CAD build for the part. Positions are in the model's coordinates, mm. A direction names the side the tool comes from. Give positions to 0.01 mm unless a question says otherwise; leave off trailing zeros. Order: outer loops, then holes, each group sorted by start corner. A loop starts at its lowest first (then second) coordinate and runs counter-clockwise, first axis right, second up.
Item 1: Band-saw the part on C-C on z = 0. Count the separate pieces of the cut face and the enclosed holes in it, plus the area to 3 significant figures.
Item 2: Wall check: L1, parallel to Z at x = -762, y = 481; L2, parallel to Y at x = -149, z = -17.5; L3, parallel to X at y = -95, z = 24.5. Give the ranges that are in metal, low to high.
Item 3: Band-saw the part on A-A on x = 762. Give the cut face in (y, z).
Item 4: Band-saw the part on B-B on y = -310. Give the cut face in (x, z).
Item 5: Two-plate mould, pull along Z, no slides. Class faces 1 (the flat face through (1016, -7, 3)), 2 (the cylindrical face through (-825.44, -476.69, 2.79)), 3 (the flat face through (-80, -449, 190.5)): released by +Z, released by -Z, zero draft, split by the parting line, or undercut.
Item 6: Band-saw the part on D-D on x = -408. Give the cut face in (y, z), plus the area to 3 significant figures.
Item 7: Which spindle directions (+Z, -Z, +X, -X, +Y, -Y) get a long thin tool onto all of the face, cutting with end or side? Do faces 4 (the flat face through (-952.5, -6, 3)), 5 (the cylindrical face through (825.44, -476.69, -2.79)). Say none if no direction does.
```python
from build123d import *

# Parameters (mm, degrees)
F0_W     = 2032
F0_H     = 1016
F0_W_2   = 1905
F0_H_2   = 889
F1_DEPTH = 190.5
F2_R     = 63.5
F3_DEPTH = 1016.001


with BuildPart() as f1:
    # F0 (on Top) → F1 (new body, symmetric)
    with BuildSketch(Plane.XY):
        Rectangle(F0_W, F0_H)
        Rectangle(F0_W_2, F0_H_2, mode=Mode.SUBTRACT)
    extrude(amount=F1_DEPTH, both=True)

    # F2 (on face) → F3 (cut, through all)
    with BuildSketch(Plane.XZ.offset(508)):
        with BuildLine():
            ThreePointArc((825.5, 0), (762, 63.5), (698.5, 0))
            ThreePointArc((698.5, 0), (762, -63.5), (825.5, 0))
        make_face()
        with BuildLine():
            ThreePointArc((63.5, 0), (0, 63.5), (-63.5, 0))
            Line((-63.5, 0), (63.5, 0))
        make_face()
        with BuildLine():
            Line((63.5, 0), (-63.5, 0))
            ThreePointArc((-63.5, 0), (0, -63.5), (63.5, 0))
        make_face()
        with Locations((-762, 0)):
            Circle(F2_R)
    extrude(amount=-F3_DEPTH, mode=Mode.SUBTRACT)


solid = f1.part
```
The answers:
1. separate pieces: 6
1. enclosed holes: 0
1. area: 323,000 mm2
2. L1: z = -190.5 to -63.5, 63.5 to 190.5
2. L2: y = -508 to -444.5, 444.5 to 508
2. L3: x = -1016 to -952.5, 952.5 to 1016
3. outline: (-508, -190.5) - (-444.5, -190.5) - (-444.5, -63.5) - (-508, -63.5) - close; (-508, 63.5) - (-444.5, 63.5) - (-444.5, 190.5) - (-508, 190.5) - close; (444.5, -190.5) - (508, -190.5) - (508, -63.5) - (444.5, -63.5) - close; (444.5, 63.5) - (508, 63.5) - (508, 190.5) - (444.5, 190.5) - close
4. outline: (-1016, -190.5) - (-952.5, -190.5) - (-952.5, 190.5) - (-1016, 190.5) - close; (952.5, -190.5) - (1016, -190.5) - (1016, 190.5) - (952.5, 190.5) - close
5. face 1: zero draft
5. face 2: undercut
5. face 3: released by +Z
6. outline: (-508, -190.5) - (-444.5, -190.5) - (-444.5, 190.5) - (-508, 190.5) - close; (444.5, -190.5) - (508, -190.5) - (508, 190.5) - (444.5, 190.5) - close
6. area: 48,400 mm2
7. face 4: +Z, -Z
7. face 5: +Y, -Y
